```python
from build123d import *

# Parameters (mm, degrees)
BOSS_EXTRUDE1_DEPTH     = 2
SCALE1_SCALE            = 2
SKETCH6_R               = 1.5
CUT_EXTRUDE2_DEPTH      = 3
SKETCH7_W               = 25
SKETCH7_H               = 3
BOSS_EXTRUDE2_DEPTH     = 15
SKETCH8_R               = 1.5
SKETCH8_W               = 16
SKETCH8_H               = 11
CUT_EXTRUDE3_DEPTH      = 18
FILLET3_R               = 3
FILLET4_R               = 3
SKETCH10_R              = 1.5
CUT_EXTRUDE4_DEPTH      = 10
CUT_EXTRUDE5_DEPTH      = 52.533558907
CUT_EXTRUDE5_DEPTH_BACK = 52.533558907
SKETCH11_R              = 44.440054466
SKETCH11_W              = 25
SKETCH11_H              = 3


with BuildPart() as part:
    # Sketch2 → Boss-Extrude1 (new body)
    with BuildSketch(Plane(origin=(0, 0, 0), x_dir=(1, 0, 0), z_dir=(0, 1, 0))):
        with BuildLine():
            Line((-17.967387551, 9.159795774), (-20.639475337, 7.15016677))
            ThreePointArc((-20.639475337, 7.15016677), (-18.649238809, 4.17439457), (-19.346117765, 0.662896123))
            ThreePointArc((-19.346117765, 0.662896123), (-19.45411943, -1.286546543), (-18.558961711, -3.021678736))
            ThreePointArc((-18.558961711, -3.021678736), (-16.421478173, -5.190969631), (-13.78312899, -6.712078584))
            ThreePointArc((-13.78312899, -6.712078584), (-13.032173848, -6.916004841), (-12.276686285, -7.102440046))
            ThreePointArc((-12.276686285, -7.102440046), (-12.194265553, -8.245293076), (-11.737308023, -9.296052821))
            ThreePointArc((-11.737308023, -9.296052821), (-10.975506649, -9.937799505), (-10.090124565, -10.394175126))
            Line((-10.090124565, -10.394175126), (-7.391598262, -11.698651137))
            Line((-7.391598262, -11.698651137), (7.391598262, -11.698651137))
            Line((7.391598262, -11.698651137), (10.090124565, -10.394175126))
            ThreePointArc((10.090124565, -10.394175126), (10.975506649, -9.937799505), (11.737308023, -9.296052821))
            ThreePointArc((11.737308023, -9.296052821), (12.194265553, -8.245293076), (12.276686285, -7.102440046))
            ThreePointArc((12.276686285, -7.102440046), (13.032173848, -6.916004841), (13.78312899, -6.712078584))
            ThreePointArc((13.78312899, -6.712078584), (16.421478173, -5.190969631), (18.558961711, -3.021678736))
            ThreePointArc((18.558961711, -3.021678736), (19.45411943, -1.286546543), (19.346117765, 0.662896123))
            ThreePointArc((19.346117765, 0.662896123), (18.649238809, 4.17439457), (20.639475337, 7.15016677))
            Line((20.639475337, 7.15016677), (17.967387551, 9.159795774))
            ThreePointArc((17.967387551, 9.159795774), (10.858325227, 7.499674132), (4.169484372, 10.424426945))
            Line((4.169484372, 10.424426945), (2.224138848, 10.424426945))
            Line((2.224138848, 10.424426945), (0.696104526, 13.114793475))
            Line((0.696104526, 13.114793475), (0, 13.358013588))
            Line((0, 13.358013588), (-0.696104526, 13.114793475))
            Line((-0.696104526, 13.114793475), (-2.224138848, 10.424426945))
            Line((-2.224138848, 10.424426945), (-4.169484372, 10.424426945))
            ThreePointArc((-4.169484372, 10.424426945), (-10.858325227, 7.499674132), (-17.967387551, 9.159795774))
        make_face()
    extrude(amount=BOSS_EXTRUDE1_DEPTH)


with BuildPart() as part_1:
    # Scale1: scaled about (0, 1, 0.242383844)
    add(part.part.scale(SCALE1_SCALE).moved(Location((0, -1, -0.242383844))))

    # Sketch6 → Cut-Extrude2 (cut)
    with BuildSketch(Plane(origin=(0, 3, 0), x_dir=(1, 0, 0), z_dir=(0, 1, 0))):
        with Locations(Location((-5.851533015, 16.28357055, 0), (0, 0, 270))):
            Circle(SKETCH6_R)
        with Locations(Location((4.151829214, 16.28357055, 0), (0, 0, 270))):
            Circle(SKETCH6_R)
    extrude(amount=-CUT_EXTRUDE2_DEPTH, mode=Mode.SUBTRACT)

    # Sketch7 → Boss-Extrude2 (add)
    with BuildSketch(Plane(origin=(0, 3, 0), x_dir=(1, 0, 0), z_dir=(0, 1, 0))):
        with Locations((0, 11.610861671)):
            Rectangle(SKETCH7_W, SKETCH7_H)
    extrude(amount=BOSS_EXTRUDE2_DEPTH)

    # Sketch8 → Cut-Extrude3 (cut)
    with BuildSketch(Plane.XY.offset(-10.110861671)):
        with Locations((-9.75, 10.917386914)):
            Circle(SKETCH8_R)
        with Locations((9.75, 10.917386914)):
            Circle(SKETCH8_R)
        with Locations((0, 10.917386914)):
            Rectangle(SKETCH8_W, SKETCH8_H)
    extrude(amount=-CUT_EXTRUDE3_DEPTH, mode=Mode.SUBTRACT)

    # Fillet3
    fillet3_edges = [part_1.edges().sort_by_distance(p)[0] for p in [
        (-12.5, 18, -11.610861671),
    ]]
    fillet(fillet3_edges, radius=FILLET3_R)

    # Fillet4
    fillet4_edges = [part_1.edges().sort_by_distance(p)[0] for p in [
        (12.5, 18, -11.610861671),
    ]]
    fillet(fillet4_edges, radius=FILLET4_R)

    # Sketch10 → Cut-Extrude4 (cut)
    with BuildSketch(Plane(origin=(0, 3, 0), x_dir=(1, 0, 0), z_dir=(0, 1, 0))):
        with Locations(Location((-0.8498519, -20.895328087, 0), (0, 0, 270))):
            Circle(SKETCH10_R)
    extrude(amount=-CUT_EXTRUDE4_DEPTH, mode=Mode.SUBTRACT)

    # Sketch11 → Cut-Extrude5 (cut, two sides: drawn at the far end of the back side and taken through both)
    with BuildSketch(Plane(origin=(0, 3, 0), x_dir=(1, 0, 0), z_dir=(0, 1, 0)).offset(-CUT_EXTRUDE5_DEPTH_BACK)):
        Circle(SKETCH11_R)
        with Locations((0, 11.610861671)):
            Rectangle(SKETCH11_W, SKETCH11_H, mode=Mode.SUBTRACT)
    extrude(amount=CUT_EXTRUDE5_DEPTH + CUT_EXTRUDE5_DEPTH_BACK, mode=Mode.SUBTRACT)


solid = part_1.part
```
Design review of the part built by this model. Coordinates are the model's own, in mm. A direction names the side the tool comes from. Coordinates: 2 decimals unless noted, no trailing zeros. Write each loop counter-clockwise with the first axis right and the second up, starting at its lowest first coordinate (ties: lowest second). Pieces come first, ordered by that corner, then holes.
1) Add section C-C (y = 10.25). Write out the cut boundary in (x, z).
2) Add section D-D (z = -11.5). Write out the cut boundary in (x, y).
3) Mouldability with a two-part tool opening along Y and no side actions: class faces 3 (the flat face through (0, 16.417, -12)), 4 (the flat face through (0, -1, -12)), 5 (the flat face through (0, 4, -10.111)) as +Y half, -Y half, draft (parallel to the pull), parting line (faces both ways), or undercut.
4) Machinability: for faces 1 (the flat face through (8, 11, -12)), 2 (the cylindrical face through (-11.64, 17.1, -11.63)), which of the approach directions +Z, -Z, +X, -X, +Y, -Y give a long, thin tool a straight path to every point of the face, cutting with its end or side? Answer none if there is none.
5) Add section A-A (y = 13.5). Write out the cut boundary in (x, z), plus the area to 3 significant figures.
6) To check wall thickness, follow L1, parallel to X at y = 11, z = -10.5; L2, parallel to Y at x = 1.5, z = -12.55; L3, parallel to X at y = 10.25, z = -11.8. State the ranges of each line that lie inside material, in increasing order.
7) Insertion check: pin 1 (2.5 mm diameter, centred on x = -9.75, y = 10.92, fed in from +Z). The pin has a flat end and moves straight along its axis. Give the tip position at first contact, or say it passes through.
8) Add section B-B (x = 2.5). Write out the cut boundary in (y, z).
Check result:
1. outline: (-12.5, -13.11) - (-11.09, -13.11) - (-11.09, -10.11) - (-12.5, -10.11) - close; (-8.41, -13.11) - (-8, -13.11) - (-8, -10.11) - (-8.41, -10.11) - close; (8, -13.11) - (8.41, -13.11) - (8.41, -10.11) - (8, -10.11) - close; (11.09, -13.11) - (12.5, -13.11) - (12.5, -10.11) - (11.09, -10.11) - close
2. outline: (-12.5, -1) - (12.5, -1) - (12.5, 15) arc R3 ccw to (9.5, 18) - (-9.5, 18) arc R3 ccw to (-12.5, 15) - close; hole circle Ø3 at (-9.75, 10.92); hole (-8, 5.42) - (8, 5.42) - (8, 16.42) - (-8, 16.42) - close; hole circle Ø3 at (9.75, 10.92)
3. face 3: undercut
3. face 4: -Y half
3. face 5: draft
4. face 1: +Z, -Z
4. face 2: +Z, -Z, -X, +Y
5. outline: (-12.5, -13.11) - (-8, -13.11) - (-8, -10.11) - (-12.5, -10.11) - close; (8, -13.11) - (12.5, -13.11) - (12.5, -10.11) - (8, -10.11) - close
5. area: 27.0 mm2
6. L1: x = -12.5 to -11.25, -8.25 to -8, 8 to 8.25, 11.25 to 12.5
6. L2: y = -1 to 5.42, 16.42 to 18
6. L3: x = -12.5 to -11.09, -8.41 to -8, 8 to 8.41, 11.09 to 12.5
7. pin 1: passes through
8. outline: (-1, -13.11) - (5.42, -13.11) - (5.42, -10.11) - (-1, -10.11) - close; (16.42, -13.11) - (18, -13.11) - (18, -10.11) - (16.42, -10.11) - close
